Here's how the part is built. I have some questions about the finished solid (model axes, mm). Face numbers are marked on the shaded views. A direction names the side the tool comes from. Give positions to 0.01 mm unless a question says otherwise; leave off trailing zeros. Order: outer loops, then holes, each group sorted by start corner. A loop starts at its lowest first (then second) coordinate and runs counter-clockwise, first axis right, second up. Notation, with made-up numbers: M -14.75,13 L -2.75,13 A29 cw -2.75,37 Z; hole C -1.5,-12.75 d7. An arc over 180 degrees is marked long. Use one line per item in the form item = value.
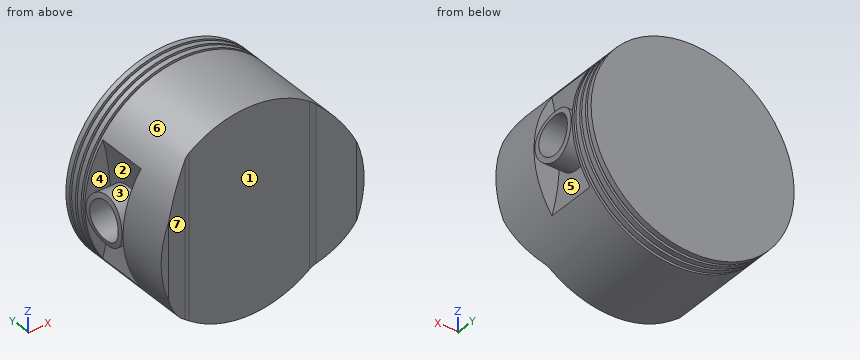
from build123d import *

# Parameters (mm, degrees)
SKETCH1_W                            = 40
SKETCH1_H                            = 50
CUT_EXTRUDE1_DEPTH                   = 55
SKETCH3_R                            = 90
CUT_EXTRUDE4_DEPTH                   = 20
BOSS_EXTRUDE1_REACH                  = 63.847
BOSS_EXTRUDE1_END_RADIUS             = 40
SKETCH4_R                            = 9.5
BOSS_EXTRUDE1_DIRECTION_2_REACH      = 63.847
BOSS_EXTRUDE1_DIRECTION_2_END_RADIUS = 40
SKETCH5_R                            = 7.5
CUT_EXTRUDE5_DEPTH                   = 55
SKETCH6_W                            = 1
SKETCH6_H                            = 1


with BuildPart() as part:
    # Sketch1 → Revolve1 (revolve)
    with BuildSketch(Plane.XY):
        with Locations((-20, 0)):
            Rectangle(SKETCH1_W, SKETCH1_H)
    revolve(axis=Axis((0, 25, 0), (0, -1, 0)))

    # Sketch2 → Cut-Extrude1 (cut, symmetric)
    with BuildSketch(Plane.XY):
        with BuildLine():
            Line((-37, -25), (-25.803847577, -18.535898385))
            ThreePointArc((-25.803847577, -18.535898385), (-24.839123758, -18.136296695), (-23.803847577, -18))
            Line((-23.803847577, -18), (23.803847577, -18))
            ThreePointArc((23.803847577, -18), (24.839123758, -18.136296695), (25.803847577, -18.535898385))
            Line((25.803847577, -18.535898385), (37, -25))
            Line((37, -25), (-37, -25))
        make_face()
    extrude(amount=CUT_EXTRUDE1_DEPTH, both=True, mode=Mode.SUBTRACT)

    # Sketch3 → Cut-Extrude4 (cut)
    with BuildSketch(Plane(origin=(0, -5, 0), x_dir=(-1, 0, 0), z_dir=(0, -1, 0))):
        with Locations((-120, 0)):
            Circle(SKETCH3_R)
        with Locations((120, 0)):
            Circle(SKETCH3_R)
    extrude(amount=-CUT_EXTRUDE4_DEPTH, mode=Mode.SUBTRACT)

    # Boss-Extrude1: up to this cylinder (the profile starts inside it)
    boss_extrude1_end = Plane(origin=(0, 5, 0), z_dir=(0, 1, 0)) * Cylinder(BOSS_EXTRUDE1_END_RADIUS, 208.694, mode=Mode.PRIVATE)
    # Sketch4 → Boss-Extrude1 (add, up to the surface)
    with BuildSketch(Plane(origin=(0, 0, 0), x_dir=(0, 0, -1), z_dir=(1, 0, 0)), mode=Mode.PRIVATE) as boss_extrude1_sk1:
        with Locations(Location((0, 5, 0), (0, 0, 180))):
            Circle(SKETCH4_R)
    boss_extrude1_tool1 = extrude(boss_extrude1_sk1.sketch, amount=BOSS_EXTRUDE1_REACH, mode=Mode.PRIVATE) & boss_extrude1_end
    add(boss_extrude1_tool1.solids().sort_by_distance((0, 5, 0))[0])

    # Boss-Extrude1 direction 2: up to this cylinder (the profile starts inside it)
    boss_extrude1_direction_2_end = Plane(origin=(0, 5, 0), z_dir=(0, 1, 0)) * Cylinder(BOSS_EXTRUDE1_DIRECTION_2_END_RADIUS, 208.694, mode=Mode.PRIVATE)
    # Sketch4 → Boss-Extrude1 direction 2 (add, up to the surface)
    with BuildSketch(Plane(origin=(0, 0, 0), x_dir=(0, 0, -1), z_dir=(1, 0, 0)), mode=Mode.PRIVATE) as boss_extrude1_direction_2_sk1:
        with Locations(Location((0, 5, 0), (0, 0, 180))):
            Circle(SKETCH4_R)
    boss_extrude1_direction_2_tool1 = extrude(boss_extrude1_direction_2_sk1.sketch, amount=-BOSS_EXTRUDE1_DIRECTION_2_REACH, mode=Mode.PRIVATE) & boss_extrude1_direction_2_end
    add(boss_extrude1_direction_2_tool1.solids().sort_by_distance((0, 5, 0))[0])

    # Sketch5 → Cut-Extrude5 (cut, symmetric)
    with BuildSketch(Plane(origin=(0, 0, 0), x_dir=(0, 0, -1), z_dir=(1, 0, 0))):
        with Locations((0, 5)):
            Circle(SKETCH5_R)
    extrude(amount=CUT_EXTRUDE5_DEPTH, both=True, mode=Mode.SUBTRACT)

    # Sketch6 → Cut-Revolve1 (revolve, cut)
    with BuildSketch(Plane.XY, mode=Mode.PRIVATE) as cut_revolve1_sk:
        with Locations((-39.5, 22.5)):
            Rectangle(SKETCH6_W, SKETCH6_H)
        with Locations((-39.5, 19.5)):
            Rectangle(SKETCH6_W, SKETCH6_H)
        with Locations((-39.5, 16.5)):
            Rectangle(SKETCH6_W, SKETCH6_H)
    revolve(cut_revolve1_sk.sketch.rotate(Axis((0, 0, 0), (0, 1, 0)), 180), axis=Axis((0, 0, 0), (0, 1, 0)), mode=Mode.SUBTRACT)


solid = part.part
Q1. On a 3-axis mill with a long thin cutter (end or side, diameter ignored), from which of +Z, -Z, +X, -X, +Y, -Y can I reach the whole of each face in a straight line? I mean the marked faces 4, 5, 6 and 7. Say none if no direction works.
Found:
face_4 = -X
face_5 = +X
face_6 = +Y, -Y
face_7 = +Z, -Z, -Y
Q2. I want a section at B-B on y = 5. Write out the boundary of the cut face in (x, z).
Found:
outline = M -39.29,-7.5 A40 ccw -38.86,-9.5 L -30.5,-9.5 A90 cw -32.92,-22.73 A40 ccw 32.92,-22.73 A90 cw 30.5,-9.5 L 38.86,-9.5 A40 ccw 39.29,-7.5 Z; M -39.29,7.5 L 39.29,7.5 A40 ccw 38.86,9.5 L 30.5,9.5 A90 cw 32.92,22.73 A40 ccw -32.92,22.73 A90 cw -30.5,9.5 L -38.86,9.5 A40 ccw Z
Q3. Thinking about a two-plate mould opening in X: for the marked faces 1, 2 and 3, which applies, +X half, -X half, draft (parallel to the pull), parting line (faces both ways), or undercut?
Found:
face_1 = undercut
face_2 = -X half
face_3 = draft
Q4. I'm going to push flat-ended pins straight in: pin 1 Ø10 at (x, z) = (-11, 30.5) entering from -Y; pin 2 Ø5 at (x, y) = (23, 1) entering from -Z; pin 3 Ø5 at (x, y) = (-5.5, -11) entering from +Z; pin 4 Ø13.5 at (y, z) = (5, 0) entering from +X. Where does each tip first touch, or does it pass through?
Found:
pin_1 = -18
pin_2 = -34.35
pin_3 = 39.89
pin_4 = through
Q5. I need wall thicknesses on L1, parallel to Y at x = -4, z = 0; L2, parallel to Y at x = 31.5, z = 2.5; L3, parallel to Z at x = -2, y = 5. Which ranges of each line are inside material? Lowest first, please.
Found:
L1 = -18 to -2.5, 12.5 to 25
L2 = -21.82 to -5, -4.17 to -2.07, 12.07 to 14.17, 15 to 25
L3 = -39.95 to -7.5, 7.5 to 39.95
